```python
from build123d import *

# Parameters (mm, degrees)
SKETCH3_R           = 4.5
BOSS_EXTRUDE1_DEPTH = 10
SKETCH4_R           = 1.6
CUT_EXTRUDE1_DEPTH  = 10
CUT_EXTRUDE2_START  = 49
SKETCH9_R           = 1.6
CUT_EXTRUDE2_DEPTH  = 49


with BuildPart() as part:
    # Sketch3 → Boss-Extrude1 (new body)
    with BuildSketch(Plane(origin=(0, 0, 0), x_dir=(1, 0, 0), z_dir=(0, 1, 0))):
        with Locations(Location((0, 0, 0), (0, 0, 270))):
            Circle(SKETCH3_R)
    extrude(amount=BOSS_EXTRUDE1_DEPTH)

    # Sketch4 → Cut-Extrude1 (cut)
    with BuildSketch(Plane.XY):
        with Locations((0, 5)):
            Circle(SKETCH4_R)
    extrude(amount=-CUT_EXTRUDE1_DEPTH, mode=Mode.SUBTRACT)

    # Sketch9 → Cut-Extrude2 (cut)
    with BuildSketch(Plane.XY.offset(CUT_EXTRUDE2_START)):
        with Locations(Location((0, 5, 0), (0, 0, 90))):
            Circle(SKETCH9_R)
    extrude(amount=-CUT_EXTRUDE2_DEPTH, mode=Mode.SUBTRACT)


solid = part.part
```
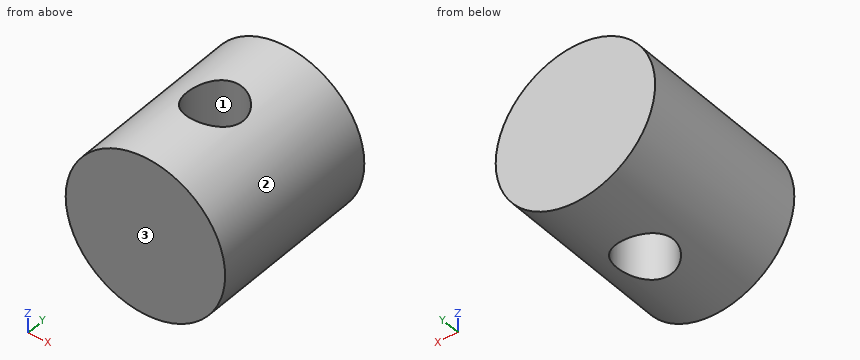
Check sheet for the modelled part. Datum: model origin and axes. Units: mm. Face numbers are marked on the shaded views. Coordinates: 2 decimals unless noted, no trailing zeros. Order: outer loops, then holes, each group sorted by start corner. A loop starts at its lowest first (then second) coordinate and runs counter-clockwise, first axis right, second up. Notation, with made-up numbers: (17, 20.5) -> (46, 20.5) arc R16 cw to (46, 33.5) -> close; hole circle Ø11 at (63, 79). An arc over 180 degrees is marked (long way). Write item = value, one per line. Start each with the question number.
1) Mould release check, pull along X, two halves, no side actions. Record for the marked faces 1, 2 and 3: +X half, -X half, draft (parallel to the pull), parting line (faces both ways), or undercut.
2) Cross-section at A-A (x = -0.25). Enter the section's corners in (y, z).
3) Cross-section at D-D (z = 2). Enter the section's corners in (x, y), then the cut area to 3 significant figures.
4) Material ranges on L1, parallel to Y at x = 0, z = 1; L2, parallel to Y at x = -1, z = 2; L3, parallel to X at y = 3.75, z = -0.75, recorded low to high.
5) Cross-section at C-C (y = 2.75). Enter the section's corners in (x, z), then the cut area to 3 significant figures.
6) Go/stop test with flat-tipped pins: P1, Ø1, axis at y = 4, z = 1.5, coming from the +X side; P2, Ø3, axis at y = 6, z = -2, coming from the -X side; P3, Ø1, axis at x = -3, y = 5.5, coming from the +Z side. Record where each tip stops, or that it passes through.
7) Cross-section at B-B (z = -4). Enter the section's corners in (x, y).
Ans:
q1.face_1 = undercut
q1.face_2 = parting line
q1.face_3 = draft
q2.outline = (0, -4.49) -> (3.42, -4.49) -> (3.42, 4.49) -> (0, 4.49) -> close; (6.58, -4.49) -> (10, -4.49) -> (10, 4.49) -> (6.58, 4.49) -> close
q3.outline = (-4.03, 0) -> (4.03, 0) -> (4.03, 10) -> (-4.03, 10) -> close; hole circle Ø3.2 at (0, 5)
q3.area = 72.6 mm²
q4.L1 = 0 to 3.4, 6.6 to 10
q4.L2 = 0 to 3.75, 6.25 to 10
q4.L3 = -4.44 to -1, 1 to 4.44
q5.outline = circle Ø9 at (0, 0)
q5.area = 63.6 mm²
q6.P1 = 4.39
q6.P2 = -4.47
q6.P3 = 3.74
q7.outline = (-2.06, 0) -> (2.06, 0) -> (2.06, 10) -> (-2.06, 10) -> close; hole circle Ø3.2 at (0, 5)
